```python
from build123d import *

# Parameters (mm, degrees)
F0_W     = 91.44
F0_H     = 40.64
F1_DEPTH = 5.08
F0_W_2   = 101.6
F0_H_2   = 50.8
F2_DEPTH = 5.08
F3_DEPTH = 10.16


with BuildPart() as f1:
    # F0 (on Top) → F1 (new body)
    with BuildSketch(Plane.XY):
        Rectangle(F0_W, F0_H)
    extrude(amount=F1_DEPTH)

    # F0 (on Top) → F2 (join)
    with BuildSketch(Plane.XY):
        Rectangle(F0_W_2, F0_H_2)
        Rectangle(F0_W, F0_H, mode=Mode.SUBTRACT)
    extrude(amount=F2_DEPTH)

    # F0 (on Top) → F3 (join)
    with BuildSketch(Plane.XY):
        Rectangle(F0_W, F0_H)
    extrude(amount=F3_DEPTH)


solid = f1.part
```
Input: part model. Units: mm. Frame: model coordinates. A direction names the side the tool comes from. Give positions to 0.01 mm unless a question says otherwise; leave off trailing zeros. Order: outer loops, then holes, each group sorted by start corner. A loop starts at its lowest first (then second) coordinate and runs counter-clockwise, first axis right, second up. Notation, with made-up numbers: (-16.5, 22) - (30.5, 22) arc R22 cw to (30.5, 45) - close; hole circle Ø8 at (86.5, 38). An arc over 180 degrees is marked (long way). Put each result on its own line as item: value.
Item 1: Ray query, L1, parallel to X at y = 15.5, z = 6; L2, parallel to Z at x = 46.5, y = -4; L3, parallel to Y at x = 13, z = 7.75. Return the intervals inside material, ascending. Write a range as from..to.
Found:
L1: x = -45.72..45.72
L2: z = 0..5.08
L3: y = -20.32..20.32
Item 2: Section query B-B, the plane y = 19. Return loops of the section in (x, z).
Found:
outline: (-50.8, 0) - (50.8, 0) - (50.8, 5.08) - (45.72, 5.08) - (45.72, 10.16) - (-45.72, 10.16) - (-45.72, 5.08) - (-50.8, 5.08) - close
Item 3: Section query C-C, the plane z = 8.75. Return loops of the section in (x, y), then the cut area to 3 significant figures.
Found:
outline: (-45.72, -20.32) - (45.72, -20.32) - (45.72, 20.32) - (-45.72, 20.32) - close
area: 3,720 mm^2
Item 4: Section query A-A, the plane x = -38.5. Return loops of the section in (y, z).
Found:
outline: (-25.4, 0) - (25.4, 0) - (25.4, 5.08) - (20.32, 5.08) - (20.32, 10.16) - (-20.32, 10.16) - (-20.32, 5.08) - (-25.4, 5.08) - close
Item 5: Access query for faces 1 (the flat face through (-1, 20.32, 8)), 2 (the flat face through (-45.72, 0, 8)), 3 (the flat face through (45.72, 0, 8)), 4 (the flat face through (-1, 0, 0)), 5 (the flat face through (-1, -20.32, 8)). Directions: +Z, -Z, +X, -X, +Y, -Y. A direction counts if a zero-diameter tool reaches every point of the face in a straight line with its end or side. Return the directions, or none.
Found:
face 1: +Z, +X, -X, +Y
face 2: +Z, -X, +Y, -Y
face 3: +Z, +X, +Y, -Y
face 4: -Z, +X, -X, +Y, -Y
face 5: +Z, +X, -X, -Y
Item 6: Contact query for flat-ended pins moving along their axis: pin 1 (2.5 mm diameter, centred on x = 6, z = 8, fed in from +Y); pin 2 (5.5 mm diameter, centred on y = -3.5, z = 8, fed in from +X); pin 3 (1.5 mm diameter, centred on y = -8, z = 7.5, fed in from -X). Output: stop coordinate, or through.
Found:
pin 1: stops at y = 20.32
pin 2: stops at x = 45.72
pin 3: stops at x = -45.72
